Verification items for this drawing (mm, ordinates from the low corner). Give positions to 0.01 mm unless a question says otherwise; leave off trailing zeros. Write each loop counter-clockwise with the first axis right and the second up, starting at its lowest first coordinate (ties: lowest second). Pieces come first, ordered by that corner, then holes. Notation, with made-up numbers: (-15, 63) -> (24, 63) arc R19 cw to (24, 89) -> close; hole circle Ø8 at (-8.75, -2). An arc over 180 degrees is marked (long way). Answer as a JSON object with one key per item and string values.
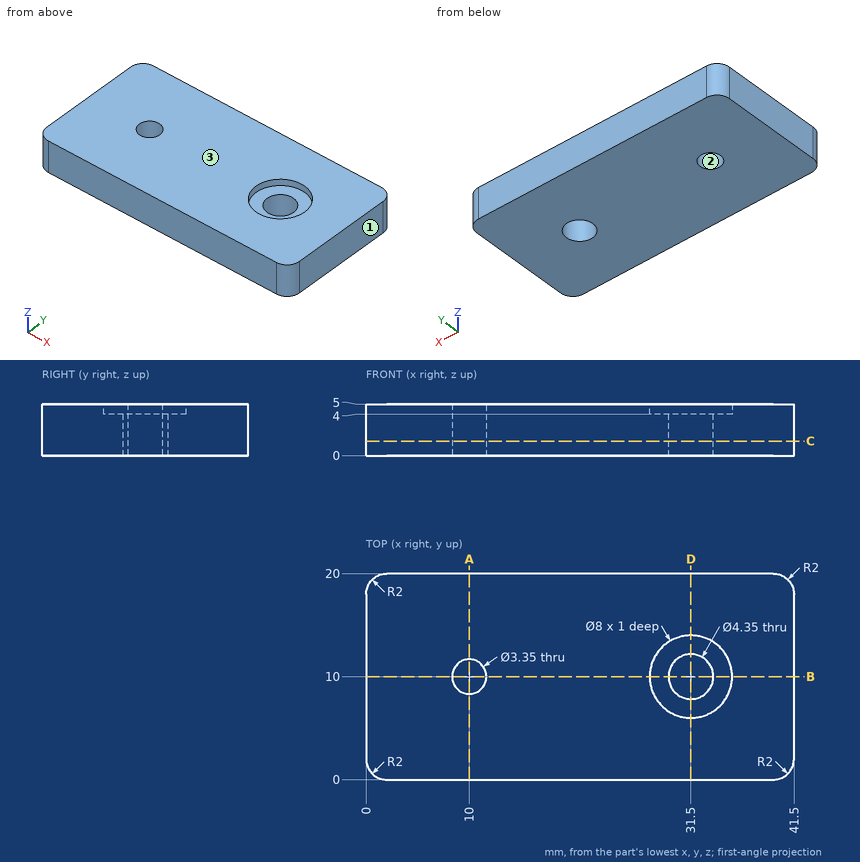
1. Sectioned sample at C-C, the plane z = 1.4. Enter the section's corners in (x, y) (3 decimals), plus the area to 3 significant figures.
Determined:
{"outline": "(0, 2) arc R2 ccw to (2, 0) -> (39.5, 0) arc R2 ccw to (41.5, 2) -> (41.5, 18) arc R2 ccw to (39.5, 20) -> (2, 20) arc R2 ccw to (0, 18) -> close; hole circle Ø3.35 at (10, 10); hole circle Ø4.35 at (31.5, 10)", "area": "803 mm^2"}
2. Go/stop test with a flat-tipped pin: P1, Ø6.5, axis at x = 31.5, y = 10, coming from the +Z side. Record where the tip stops, or that it passes through.
Determined:
{"P1": "z = 4"}
3. Scan lines: L1, parallel to Y at x = 10, z = 1.9 (3 decimals); L2, parallel to X at y = 8.5, z = 1 (3 decimals); L3, parallel to Y at x = 31.5, z = 4.85. Record each from-to range of solid material in increasing order. Write a range as [from, to].
Determined:
{"L1": "[0, 8.325], [11.675, 20]", "L2": "[0, 9.255], [10.745, 29.925], [33.075, 41.5]", "L3": "[0, 6], [14, 20]"}
4. Mould release check, pull along X, two halves, no side actions. Record for the marked faces 1, 2 and 3: released by +X, released by -X, zero draft, split by the parting line, or undercut.
Determined:
{"face 1": "released by +X", "face 2": "undercut", "face 3": "zero draft"}
5. Sectioned sample at D-D, the plane x = 31.5. Enter the section's corners in (y, z) (3 decimals).
Determined:
{"outline": "(0, 0) -> (7.825, 0) -> (7.825, 4) -> (6, 4) -> (6, 5) -> (0, 5) -> close; (12.175, 0) -> (20, 0) -> (20, 5) -> (14, 5) -> (14, 4) -> (12.175, 4) -> close"}
6. Sectioned sample at B-B, the plane y = 10. Enter the section's corners in (x, z) (3 decimals).
Determined:
{"outline": "(0, 0) -> (8.325, 0) -> (8.325, 5) -> (0, 5) -> close; (11.675, 0) -> (29.325, 0) -> (29.325, 4) -> (27.5, 4) -> (27.5, 5) -> (11.675, 5) -> close; (33.675, 0) -> (41.5, 0) -> (41.5, 5) -> (35.5, 5) -> (35.5, 4) -> (33.675, 4) -> close"}
7. Sectioned sample at A-A, the plane x = 10. Enter the section's corners in (y, z) (3 decimals), plus the area to 4 significant figures.
Determined:
{"outline": "(0, 0) -> (8.325, 0) -> (8.325, 5) -> (0, 5) -> close; (11.675, 0) -> (20, 0) -> (20, 5) -> (11.675, 5) -> close", "area": "83.25 mm^2"}
